Work out the finished part from the listing and answer in its coordinate system (mm). Coordinates: 2 decimals unless noted, no trailing zeros. Write each loop counter-clockwise with the first axis right and the second up, starting at its lowest first coordinate (ties: lowest second). Pieces come first, ordered by that corner, then holes. Notation, with made-up numbers: (89.25, 39) - (99.25, 39) arc R18 cw to (99.25, 56) - close; hole circle Ø5 at (5, 71). An arc over 180 degrees is marked (long way). Use CSV: the item, a comma, the result in double quotes. Start each with the question number.
from build123d import *

# Parameters (mm, degrees)
SKETCH1_W           = 100
SKETCH1_H           = 100
SKETCH1_R           = 19
SKETCH1_R_2         = 16.5
BOSS_EXTRUDE1_DEPTH = 10


with BuildPart() as part:
    # Sketch1 → Boss-Extrude1 (new body)
    # profile 1 of 2: a face of its own
    with BuildSketch(Plane(origin=(0, 0, 0), x_dir=(1, 0, 0), z_dir=(0, 1, 0))):
        Rectangle(SKETCH1_W, SKETCH1_H)
        Circle(SKETCH1_R, mode=Mode.SUBTRACT)
    # profile 2 of 2: a face of its own
    with BuildSketch(Plane(origin=(0, 0, 0), x_dir=(1, 0, 0), z_dir=(0, 1, 0))):
        Circle(SKETCH1_R)
        with Locations(Location((0, 0, 0), (0, 0, 270))):
            Circle(SKETCH1_R_2, mode=Mode.SUBTRACT)
    extrude(amount=BOSS_EXTRUDE1_DEPTH)


solid = part.part
Item 1: A cutting plane is placed at C-C (y = 8.75). Determine the outline of the cut face in (x, z), then the cut area to 3 significant figures.
Item 2: A cutting plane is placed at B-B (x = 0). Determine the outline of the cut face in (y, z), then the cut area to 3 significant figures.
Item 3: Straight lines are drawn through the part: probe 1 along X at (y, z) = (7, 0); probe 2 along X at (y, z) = (4.5, -15); probe 3 along Z at (x, y) = (1, 3.5). For each, find the intervals that lie inside material, in ascending order. Write a range as [from, to].
Item 4: Determine the mould class of faces 1 (the face through (-12, 10, -12)), 2 (the face through (-1, 5, 50)), 3 (the face through (-16.108, 4.93, -3.577)) for opening direction Z: +Z half, -Z half, draft (parallel to the pull), parting line (faces both ways), or undercut.
Item 5: A cutting plane is placed at A-A (z = 0). Determine the outline of the cut face in (x, y).
Calculated:
1,outline,"(-50, -50) - (50, -50) - (50, 50) - (-50, 50) - close; hole circle Ø33 at (0, 0)"
1,area,"9,140 mm²"
2,outline,"(0, -50) - (10, -50) - (10, -16.5) - (0, -16.5) - close; (0, 16.5) - (10, 16.5) - (10, 50) - (0, 50) - close"
2,area,"670 mm²"
3,probe 1,"x = [-50, -16.5], [16.5, 50]"
3,probe 2,"x = [-50, -6.87], [6.87, 50]"
3,probe 3,"z = [-50, -16.47], [16.47, 50]"
4,face 1,"draft"
4,face 2,"+Z half"
4,face 3,"undercut"
5,outline,"(-50, 0) - (-16.5, 0) - (-16.5, 10) - (-50, 10) - close; (16.5, 0) - (50, 0) - (50, 10) - (16.5, 10) - close"
